Can you work these out from the drawing? Everything is in mm from the part's minimum corner. A direction names the side the tool comes from. Round coordinates to 2 decimals unless told otherwise and drop trailing zeros. Order: outer loops, then holes, each group sorted by start corner. A loop starts at its lowest first (then second) coordinate and runs counter-clockwise, first axis right, second up. Notation, with made-up numbers: M 81.25,20.25 L 100.25,20.25 A9 ccw 100.25,37.25 Z; hole C 76,69.25 d2. An arc over 180 degrees is marked long. Answer as a JSON object with one key per item and string values. Group by question number.
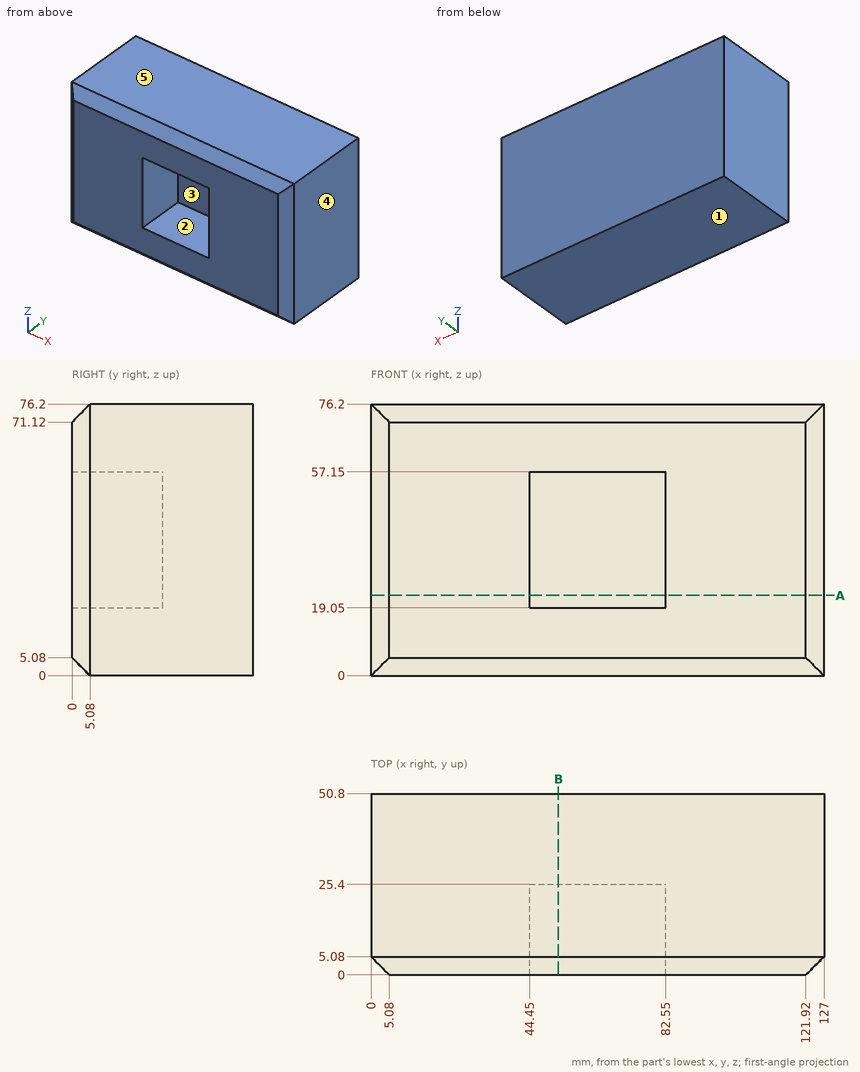
Item 1: I need wall thicknesses on line 1 (Z direction, x = 76.5, y = 21); line 2 (X direction, y = 13, z = 48); line 3 (Y direction, x = 67.5, z = 47). Which ranges of each line are inside material? Lowest first, please.
Item 2: Suppose I cut it at B-B, the plane x = 52.5. Write out the boundary of the cut face in (y, z), and give its area (3 significant figures).
Item 3: Suppose I cut it at A-A, the plane z = 22.5. Write out the boundary of the cut face in (x, y), and give its area (3 significant figures).
Item 4: If we mould it in two halves opening along Z, with no side actions, what happens to the marked faces 3, 4 and 5? For each: +Z half, -Z half, draft (parallel to the pull), parting line (faces both ways), or undercut.
Item 5: On a 3-axis mill with a long thin cutter (end or side, diameter ignored), from which of +Z, -Z, +X, -X, +Y, -Y can I reach the whole of each face in a straight line? I mean the marked faces 1 and 2. Say none if no direction works.
Computed:
{
 "1": {"line 1": "z = 0 to 19.05, 57.15 to 76.2", "line 2": "x = 0 to 44.45, 82.55 to 127", "line 3": "y = 25.4 to 50.8"},
 "2": {"outline": "M 0,5.08 L 5.08,0 L 50.8,0 L 50.8,76.2 L 5.08,76.2 L 0,71.12 L 0,57.15 L 25.4,57.15 L 25.4,19.05 L 0,19.05 Z", "area": "2,880 mm^2"},
 "3": {"outline": "M 0,5.08 L 5.08,0 L 44.45,0 L 44.45,25.4 L 82.55,25.4 L 82.55,0 L 121.92,0 L 127,5.08 L 127,50.8 L 0,50.8 Z", "area": "5,460 mm^2"},
 "4": {"face 3": "undercut", "face 4": "draft", "face 5": "+Z half"},
 "5": {"face 1": "-Z, +X, -X, +Y, -Y", "face 2": "-Y"}
}
